Here's how the part is built. I have some questions about the finished solid (model axes, mm). Face numbers are marked on the shaded views. A direction names the side the tool comes from. Round coordinates to 2 decimals unless told otherwise and drop trailing zeros. Write each loop counter-clockwise with the first axis right and the second up, starting at its lowest first coordinate (ties: lowest second). Pieces come first, ordered by that corner, then holes. Notation, with made-up numbers: (66, -38.5) -> (102, -38.5) arc R24 cw to (102, -22.5) -> close; hole circle Ø7 at (32, 85). An arc over 180 degrees is marked (long way). Answer as CSV lines item,"result".
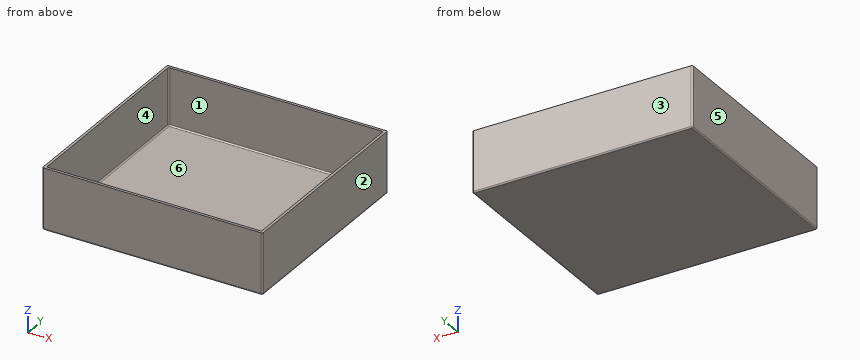
from build123d import *

# Parameters (mm, degrees)
F0_W     = 83
F0_H     = 78
F0_W_2   = 81
F0_H_2   = 76
F1_DEPTH = 23
F2_DEPTH = 1.5
F3_R     = 0.5
F4_R     = 0.5


with BuildPart() as f1:
    # F0 (on Top) → F1 (new body)
    with BuildSketch(Plane.XY):
        Rectangle(F0_W, F0_H)
        Rectangle(F0_W_2, F0_H_2, mode=Mode.SUBTRACT)
    extrude(amount=F1_DEPTH)

    # F0 (on Top) → F2 (join)
    with BuildSketch(Plane.XY):
        Rectangle(F0_W_2, F0_H_2)
    extrude(amount=F2_DEPTH)

    # F3
    f3_edges = [f1.edges().sort_by_distance(p)[0] for p in [
        (0, -39, 0),
        (-41.5, 0, 0),
        (0, 39, 0),
        (41.5, 0, 0),
        (-41.5, -39, 11.5),
        (41.5, -39, 11.5),
        (-41.5, 39, 11.5),
        (41.5, 39, 11.5),
    ]]
    fillet(f3_edges, radius=F3_R)

    # F4
    f4_edges = [f1.edges().sort_by_distance(p)[0] for p in [
        (40.5, 38, 12.25),
        (0, 38, 1.5),
        (40.5, 0, 1.5),
        (-40.5, 38, 12.25),
        (-40.5, 0, 1.5),
        (40.5, -38, 12.25),
        (0, -38, 1.5),
        (-40.5, -38, 12.25),
    ]]
    fillet(f4_edges, radius=F4_R)


solid = f1.part
Item 1: Suppose I cut it at B-B, the plane x = 31. List the corners of the cut face in (y, z) for me.
Results found:
outline,"(-39, 0.5) arc R0.5 ccw to (-38.5, 0) -> (38.5, 0) arc R0.5 ccw to (39, 0.5) -> (39, 23) -> (38, 23) -> (38, 2) arc R0.5 cw to (37.5, 1.5) -> (-37.5, 1.5) arc R0.5 cw to (-38, 2) -> (-38, 23) -> (-39, 23) -> close"
Item 2: Will this pin go through, and if not, where does the flat tip stop? pin 1 (10 mm diameter, centred on x = -25.5, y = 10.5, fed in from +Z).
Results found:
pin 1,"stops at z = 1.5"
Item 3: If we mould it in two halves opening along Y, with no side actions, what happens to the marked faces 3, 4, 5 and 6? For each: pulls with the +Y half, pulls with the -Y half, needs draft (parallel to the pull), parting line crosses it, or undercut.
Results found:
face 3,"pulls with the +Y half"
face 4,"undercut"
face 5,"needs draft"
face 6,"undercut"
Item 4: Suppose I cut it at C-C, the plane y = -21.5. List the corners of the cut face in (x, z) for me, then the cut area to 4 significant figures.
Results found:
outline,"(-41.5, 0.5) arc R0.5 ccw to (-41, 0) -> (41, 0) arc R0.5 ccw to (41.5, 0.5) -> (41.5, 23) -> (40.5, 23) -> (40.5, 2) arc R0.5 cw to (40, 1.5) -> (-40, 1.5) arc R0.5 cw to (-40.5, 2) -> (-40.5, 23) -> (-41.5, 23) -> close"
area,"167.5 mm²"
Item 5: I need wall thicknesses on L1, parallel to X at y = 36.5, z = 13.75; L2, parallel to Y at x = 31.5, z = 12.5; L3, parallel to Z at x = -21, y = -18. Which ranges of each line are inside material? Lowest first, please.
Results found:
L1,"x = -41.5 to -40.5, 40.5 to 41.5"
L2,"y = -39 to -38, 38 to 39"
L3,"z = 0 to 1.5"
Item 6: Suppose I cut it at A-A, the plane z = 18.5. List the corners of the cut face in (x, y) for me.
Results found:
outline,"(-41.5, -38.5) arc R0.5 ccw to (-41, -39) -> (41, -39) arc R0.5 ccw to (41.5, -38.5) -> (41.5, 38.5) arc R0.5 ccw to (41, 39) -> (-41, 39) arc R0.5 ccw to (-41.5, 38.5) -> close; hole (-40.5, -37.5) arc R0.5 ccw to (-40, -38) -> (40, -38) arc R0.5 ccw to (40.5, -37.5) -> (40.5, 37.5) arc R0.5 ccw to (40, 38) -> (-40, 38) arc R0.5 ccw to (-40.5, 37.5) -> close"
Item 7: For the marked faces 1 and 2, which set-ups out of +Z, -Z, +X, -X, +Y, -Y let a thin tool reach every point of the face, with its end or its side?
Results found:
face 1,"+Z"
face 2,"+Z, -Z, +X, +Y, -Y"
